Source: CAD feature listing. Evaluate the final solid. Frame: model axes, mm. A direction names the side the tool comes from. Give positions to 0.01 mm unless a question says otherwise; leave off trailing zeros. Order: outer loops, then holes, each group sorted by start corner. A loop starts at its lowest first (then second) coordinate and runs counter-clockwise, first axis right, second up. Notation, with made-up numbers: (34.25, -6.5) -> (88.25, -6.5) arc R8 cw to (88.25, 8.5) -> close; hole circle Ø6 at (10.25, -36). An arc over 180 degrees is marked (long way). Answer in a Markdown table with one row per item.
```python
from build123d import *

# Parameters (mm, degrees)
SKETCH_1_R      = 2.65
SKETCH_1_W      = 12
SKETCH_1_H      = 67.337004634
SKETCH_1_H_2    = 67.362830637
EXTRUDE_1_DEPTH = 5
FILLET_1_R      = 3


with BuildPart() as part:
    # 草图1 → 凸台-拉伸1 (new body)
    with BuildSketch(Plane.XY):
        with BuildLine():
            Line((-10, 80), (-10, -80))
            ThreePointArc((-10, -80), (0, -90), (10, -80))
            Line((10, -80), (10, 80))
            ThreePointArc((10, 80), (0, 90), (-10, 80))
        make_face()
        with Locations((0, 80)):
            Circle(SKETCH_1_R, mode=Mode.SUBTRACT)
        with Locations((0, -80)):
            Circle(SKETCH_1_R, mode=Mode.SUBTRACT)
        with Locations((0.111968731, 38.831497683)):
            Rectangle(SKETCH_1_W, SKETCH_1_H, mode=Mode.SUBTRACT)
        with Locations((0.111968731, -38.818584681)):
            Rectangle(SKETCH_1_W, SKETCH_1_H_2, mode=Mode.SUBTRACT)
    extrude(amount=EXTRUDE_1_DEPTH)

    # 圆角1
    fillet_1_edges = [part.edges().sort_by_distance(p)[0] for p in [
        (-5.888031269, 5.162995366, 2.5),
        (6.111968731, 5.162995366, 2.5),
        (6.111968731, 72.5, 2.5),
        (-5.888031269, 72.5, 2.5),
        (-5.888031269, -5.137169363, 2.5),
        (-5.888031269, -72.5, 2.5),
        (6.111968731, -72.5, 2.5),
        (6.111968731, -5.137169363, 2.5),
    ]]
    fillet(fillet_1_edges, radius=FILLET_1_R)


solid = part.part
```
(1) First-contact query: pin 1 Ø3 at (x, z) = (-2, 4) entering from +Y; pin 2 Ø7 at (x, y) = (0, 80) entering from -Z; pin 3 Ø3 at (x, z) = (-5.5, 2.5) entering from +Y; pin 4 Ø1 at (x, z) = (-3, 1) entering from +Y. Flat tips, straight axial feed; report the tip coordinate or a pass-through.
A:
| item | result |
|---|---|
| pin 1 | stops at y = 89.99 |
| pin 2 | stops at z = 0 |
| pin 3 | stops at y = 89.17 |
| pin 4 | stops at y = 89.68 |
(2) Access query for faces 1 (the flat face through (10, -1, 2)), 2 (the cylindrical face through (5.256, -6.039, 2.535)). Directions: +Z, -Z, +X, -X, +Y, -Y. A direction counts if a zero-diameter tool reaches every point of the face in a straight line with its end or side. Return the directions, or none.
A:
| item | result |
|---|---|
| face 1 | +Z, -Z, +X, +Y, -Y |
| face 2 | +Z, -Z |
(3) Section query A-A (x = 0). Return the cut outline in (y, z).
A:
| item | result |
|---|---|
| outline | (-90, 0) -> (-82.65, 0) -> (-82.65, 5) -> (-90, 5) -> close; (-77.35, 0) -> (-72.5, 0) -> (-72.5, 5) -> (-77.35, 5) -> close; (-5.14, 0) -> (5.16, 0) -> (5.16, 5) -> (-5.14, 5) -> close; (72.5, 0) -> (77.35, 0) -> (77.35, 5) -> (72.5, 5) -> close; (82.65, 0) -> (90, 0) -> (90, 5) -> (82.65, 5) -> close |
(4) Pull-direction query (Y, two-part tool) for faces 3 (the cylindrical face through (0, 90, 2)), 4 (the cylindrical face through (-4.99, 6.02, 2.54)), 5 (the flat face through (-10, 1, 2)), 6 (the cylindrical face through (0, -90, 2)); classes: +Y half, -Y half, draft (parallel to the pull), parting line (faces both ways), or undercut.
A:
| item | result |
|---|---|
| face 3 | +Y half |
| face 4 | undercut |
| face 5 | draft |
| face 6 | -Y half |
(5) Section query D-D (x = -8.5). Return the cut outline in (y, z).
A:
| item | result |
|---|---|
| outline | (-85.27, 0) -> (85.27, 0) -> (85.27, 5) -> (-85.27, 5) -> close |
(6) Section query C-C (z = 2). Return the cut outline in (x, y).
A:
| item | result |
|---|---|
| outline | (-10, -80) arc R10 ccw to (10, -80) -> (10, 80) arc R10 ccw to (-10, 80) -> close; hole (-5.89, -69.5) arc R3 ccw to (-2.89, -72.5) -> (3.11, -72.5) arc R3 ccw to (6.11, -69.5) -> (6.11, -8.14) arc R3 ccw to (3.11, -5.14) -> (-2.89, -5.14) arc R3 ccw to (-5.89, -8.14) -> close; hole (-5.89, 8.16) arc R3 ccw to (-2.89, 5.16) -> (3.11, 5.16) arc R3 ccw to (6.11, 8.16) -> (6.11, 69.5) arc R3 ccw to (3.11, 72.5) -> (-2.89, 72.5) arc R3 ccw to (-5.89, 69.5) -> close; hole circle Ø5.3 at (0, -80); hole circle Ø5.3 at (0, 80) |
(7) Ray query, probe 1 along Y at (x, z) = (0, 2.15); probe 2 along X at (y, z) = (36.5, 1.45); probe 3 along Y at (x, z) = (-5.25, 0.5). Return the intervals inside material, ascending.
A:
| item | result |
|---|---|
| probe 1 | y = -90 to -82.65, -77.35 to -72.5, -5.14 to 5.16, 72.5 to 77.35, 82.65 to 90 |
| probe 2 | x = -10 to -5.89, 6.11 to 10 |
| probe 3 | y = -88.51 to -71.35, -6.29 to 6.31, 71.35 to 88.51 |
(8) Section query B-B (y = -30). Return the cut outline in (x, z).
A:
| item | result |
|---|---|
| outline | (-10, 0) -> (-5.89, 0) -> (-5.89, 5) -> (-10, 5) -> close; (6.11, 0) -> (10, 0) -> (10, 5) -> (6.11, 5) -> close |
